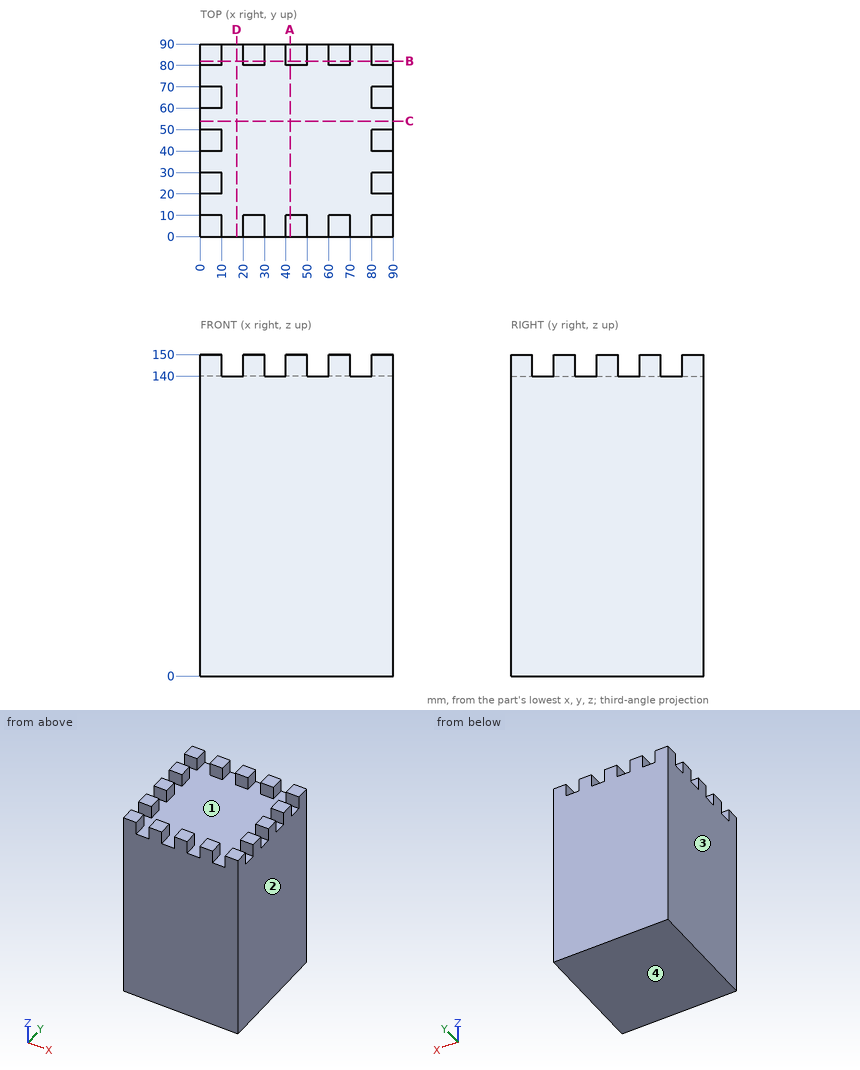
Input: dimensioned drawing with shaded views. Units: mm. Origin: part minimum x, y, z. Coordinates: 2 decimals unless noted, no trailing zeros. Order: outer loops, then holes, each group sorted by start corner. A loop starts at its lowest first (then second) coordinate and runs counter-clockwise, first axis right, second up.
1. Ray query, line 1 along Z through (x, y) = (51, 36). Return the intervals inside material, ascending.
Checked values:
line 1: z = 0 to 140
2. Cut plane A-A, the plane x = 42. Return loops of the section in (y, z).
Checked values:
outline: (0, 0) - (90, 0) - (90, 150) - (80, 150) - (80, 140) - (10, 140) - (10, 150) - (0, 150) - close
3. Cut plane B-B, the plane y = 82. Return loops of the section in (x, z).
Checked values:
outline: (0, 0) - (90, 0) - (90, 150) - (80, 150) - (80, 140) - (70, 140) - (70, 150) - (60, 150) - (60, 140) - (50, 140) - (50, 150) - (40, 150) - (40, 140) - (30, 140) - (30, 150) - (20, 150) - (20, 140) - (10, 140) - (10, 150) - (0, 150) - close
4. Draft query along X for the marked faces 1, 2, 3 and 4. Return one class per face: +X half, -X half, draft (parallel to the pull), parting line (faces both ways), or undercut.
Checked values:
face 1: undercut
face 2: +X half
face 3: -X half
face 4: draft
5. Cut plane C-C, the plane y = 54. Return loops of the section in (x, z), plus the area to 3 significant figures.
Checked values:
outline: (0, 0) - (90, 0) - (90, 140) - (0, 140) - close
area: 12,600 mm2
